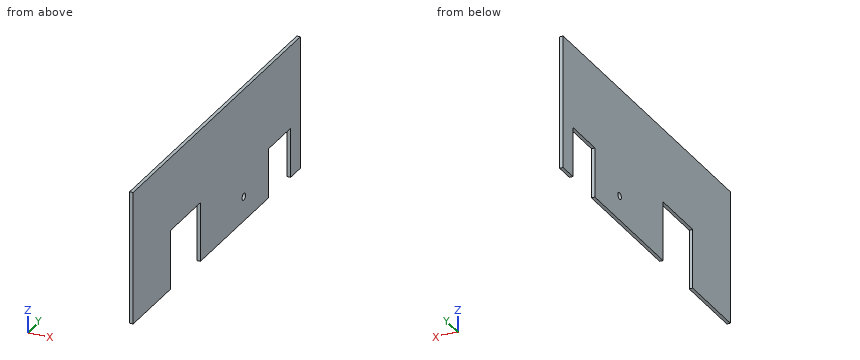
from build123d import *

# Parameters (mm, degrees)
SKETCH_1_W          = 95
SKETCH_1_H          = 38.85
EXTRUDE_1_DEPTH     = 0.5
SKETCH_2_W          = 38.85
SKETCH_2_H          = 95
EXTRUDE_2_DEPTH     = 0.5
SKETCH_3_W          = 20.065150591
SKETCH_3_H          = 12.517385588
CUT_EXTRUDE_1_DEPTH = 3
SKETCH_4_W          = 23.07389694
SKETCH_4_H          = 16.832919213
CUT_EXTRUDE_2_DEPTH = 3
SKETCH_5_R          = 0.973496531
CUT_EXTRUDE_3_DEPTH = 3


with BuildPart() as part:
    # Эскиз1 → Бобышка-Вытянуть1 (new body)
    with BuildSketch(Plane(origin=(0.5, 0, 0), x_dir=(0, -1, 0), z_dir=(-1, 0, 0))):
        with Locations((-53.35, 22.825)):
            Rectangle(SKETCH_1_W, SKETCH_1_H)
    extrude(amount=-EXTRUDE_1_DEPTH)

    # Эскиз2 → Бобышка-Вытянуть2 (add)
    with BuildSketch(Plane.ZY.offset(-0.5)):
        with Locations((22.825, 53.35)):
            Rectangle(SKETCH_2_W, SKETCH_2_H)
    extrude(amount=EXTRUDE_2_DEPTH)

    # Эскиз3 → Вырез-Вытянуть1 (cut)
    with BuildSketch(Plane.ZY):
        with Locations((7.88603419, 89.086980773)):
            Rectangle(SKETCH_3_W, SKETCH_3_H)
    extrude(amount=-CUT_EXTRUDE_1_DEPTH, mode=Mode.SUBTRACT)

    # Эскиз4 → Вырез-Вытянуть2 (cut)
    with BuildSketch(Plane.ZY):
        with Locations((9.208796156, 35.637729194)):
            Rectangle(SKETCH_4_W, SKETCH_4_H)
    extrude(amount=-CUT_EXTRUDE_2_DEPTH, mode=Mode.SUBTRACT)

    # Эскиз5 → Вырез-Вытянуть3 (cut)
    with BuildSketch(Plane.ZY):
        with Locations((10.527030872, 68.763270983)):
            Circle(SKETCH_5_R)
    extrude(amount=-CUT_EXTRUDE_3_DEPTH, mode=Mode.SUBTRACT)


solid = part.part
The listing builds one solid part. Answer for the finished solid, in the listing's coordinates (mm). Coordinates: 2 decimals unless noted, no trailing zeros. Write each loop counter-clockwise with the first axis right and the second up, starting at its lowest first coordinate (ties: lowest second). Pieces come first, ordered by that corner, then holes. Notation, with made-up numbers: M 4.25,77.25 L 63.25,77.25 A20 ccw 63.25,96.25 Z; hole C 53.5,22 d2. An arc over 180 degrees is marked long. Put each result on its own line as item: value. Start each with the question number.
1. Consider line 1 (Y direction, x = 0.75, z = 15); line 2 (Y direction, x = 0.7, z = 11); line 3 (Y direction, x = 0.9, z = 20). Determine where each line is inside the solid, lowest interval first. Write a range as from..to.
2. A cutting plane is placed at A-A on z = 7. Write down the section's boundary in (x, y).
3. A cutting plane is placed at B-B on x = 0.5. Write down the section's boundary in (y, z).
Resolved:
1. line 1: y = 5.85..27.22, 44.05..82.83, 95.35..100.85
1. line 2: y = 5.85..27.22, 44.05..67.91, 69.61..82.83, 95.35..100.85
1. line 3: y = 5.85..27.22, 44.05..100.85
2. outline: M 0,5.85 L 1,5.85 L 1,27.22 L 0,27.22 Z; M 0,44.05 L 1,44.05 L 1,82.83 L 0,82.83 Z; M 0,95.35 L 1,95.35 L 1,100.85 L 0,100.85 Z
3. outline: M 5.85,3.4 L 27.22,3.4 L 27.22,20.75 L 44.05,20.75 L 44.05,3.4 L 82.83,3.4 L 82.83,17.92 L 95.35,17.92 L 95.35,3.4 L 100.85,3.4 L 100.85,42.25 L 5.85,42.25 Z; hole C 68.76,10.53 d1.95
